Could you check a few things on this model? Use its own coordinates, in mm. A direction names the side the tool comes from. Round coordinates to 2 decimals unless told otherwise and drop trailing zeros. Loops run counter-clockwise (first coordinate to the right, second up) from the corner with the lowest first, then second, coordinate; pieces in that order, holes last. Notation, with made-up numbers: (86.25, 83.25) -> (122.25, 83.25) arc R17 ccw to (122.25, 89.25) -> close; hole circle Ø1 at (24.25, -36). An arc over 180 degrees is marked (long way). One line per item, written item: value.
from build123d import *

# Parameters (mm, degrees)
F1_DEPTH = 25.4
F2_R     = 4.7625
F3_DEPTH = 12.701
F5_DEPTH = 12.7
F6_R     = 1.5875
F7_DEPTH = 38.101
F8_R     = 5.08
F9_R     = 12.7
F10_R    = 2.032


with BuildPart() as f1:
    # F0 (on Front) → F1 (new body, symmetric)
    with BuildSketch(Plane.XZ):
        with BuildLine():
            Line((-53.975, 0), (-31.75, 0))
            ThreePointArc((-31.75, 0), (-31.0802754355, 6.4868311871), (-29.099355663, 12.7))
            Line((-29.099355663, 12.7), (-53.975, 12.7))
            Line((-53.975, 12.7), (-53.975, 0))
        make_face()
        with BuildLine():
            ThreePointArc((29.099355663, 12.7), (31.0802754355, 6.4868311871), (31.75, 0))
            Line((31.75, 0), (53.975, 0))
            Line((53.975, 0), (53.975, 38.1))
            Line((53.975, 38.1), (41.275, 38.1))
            Line((41.275, 38.1), (41.275, 12.7))
            Line((41.275, 12.7), (29.099355663, 12.7))
        make_face()
        with BuildLine():
            ThreePointArc((-14.1990316571, 12.7), (0, 19.05), (14.1990316571, 12.7))
            Line((14.1990316571, 12.7), (29.099355663, 12.7))
            ThreePointArc((29.099355663, 12.7), (0, 31.75), (-29.099355663, 12.7))
            Line((-29.099355663, 12.7), (-14.1990316571, 12.7))
        make_face()
        with BuildLine():
            ThreePointArc((14.1990316571, 12.7), (17.7959834382, 6.7974608102), (19.05, 0))
            Line((19.05, 0), (31.75, 0))
            ThreePointArc((31.75, 0), (31.0802754355, 6.4868311871), (29.099355663, 12.7))
            Line((29.099355663, 12.7), (14.1990316571, 12.7))
        make_face()
        with BuildLine():
            Line((-31.75, 0), (-19.05, 0))
            ThreePointArc((-19.05, 0), (-17.7959834382, 6.7974608102), (-14.1990316571, 12.7))
            Line((-14.1990316571, 12.7), (-29.099355663, 12.7))
            ThreePointArc((-29.099355663, 12.7), (-31.0802754355, 6.4868311871), (-31.75, 0))
        make_face()
    extrude(amount=F1_DEPTH, both=True)

    # F2 (on face) → F3 (cut, through all)
    with BuildSketch(Plane.XY.offset(12.7)):
        with Locations((-41.275, 11.3)):
            Circle(F2_R)
        with Locations((-41.275, -11.3)):
            Circle(F2_R)
    extrude(amount=-F3_DEPTH, mode=Mode.SUBTRACT)

    # F4 (on face) → F5 (cut, through all)
    with BuildSketch(Plane.YZ.offset(53.975)):
        with BuildLine():
            Line((6.5, 38.1), (-6.5, 38.1))
            Line((-6.5, 38.1), (-6.5, 25))
            ThreePointArc((-6.5, 25), (0, 31.5), (6.5, 25))
            Line((6.5, 25), (6.5, 38.1))
        make_face()
        with BuildLine():
            ThreePointArc((6.5, 25), (0, 31.5), (-6.5, 25))
            Line((-6.5, 25), (6.5, 25))
        make_face()
        with BuildLine():
            Line((6.5, 25), (-6.5, 25))
            ThreePointArc((-6.5, 25), (0, 18.5), (6.5, 25))
        make_face()
    extrude(amount=-F5_DEPTH, mode=Mode.SUBTRACT)

    # F6 (on face) → F7 (cut, through all)
    with BuildSketch(Plane(origin=(0, 0, 0), x_dir=(1, 0, 0), z_dir=(0, 0, -1))):
        Circle(F6_R)
    extrude(amount=-F7_DEPTH, mode=Mode.SUBTRACT)

    # F8
    f8_edges = [f1.edges().sort_by_distance(p)[0] for p in [
        (47.625, -25.4, 38.1),
        (47.625, 25.4, 38.1),
        (29.099356, 0, 12.7),
        (41.275, 0, 12.7),
        (-29.099356, 0, 12.7),
    ]]
    fillet(f8_edges, radius=F8_R)

    # F9
    f9_edges = [f1.edges().sort_by_distance(p)[0] for p in [
        (-53.975, 25.4, 6.35),
        (-53.975, -25.4, 6.35),
    ]]
    fillet(f9_edges, radius=F9_R)

    # F10
    f10_edges = [f1.edges().sort_by_distance(p)[0] for p in [
        (-36.7645, -25.4, 12.7),
    ]]
    fillet(f10_edges, radius=F10_R)


solid = f1.part
(1) If we section it at D-D, the plane y = 4: Please give me the cut outline in (x, z) (3 decimals).
Recorded:
outline: (-53.975, 0) -> (-19.05, 0) arc R19.05 cw to (19.05, 0) -> (53.975, 0) -> (53.975, 19.877) -> (41.275, 19.877) -> (41.275, 17.78) arc R5.08 cw to (36.195, 12.7) -> (32.254, 12.7) arc R5.08 cw to (27.805, 15.328) arc R31.75 ccw to (-27.805, 15.328) arc R5.08 cw to (-32.254, 12.7) -> (-51.943, 12.7) arc R2.032 ccw to (-53.975, 10.668) -> close
(2) If we section it at B-B, the plane z = 4: Please give me the cut outline in (x, y) (1 decimal), then the cut area to 3 significant figures.
Recorded:
outline: (-54, -12.7) arc R12.7 ccw to (-41.3, -25.4) -> (-18.6, -25.4) -> (-18.6, 25.4) -> (-41.3, 25.4) arc R12.7 ccw to (-54, 12.7) -> close; (18.6, -25.4) -> (54, -25.4) -> (54, 25.4) -> (18.6, 25.4) -> close; hole circle Ø9.5 at (-41.3, -11.3); hole circle Ø9.5 at (-41.3, 11.3)
area: 3,380 mm²
(3) If we section it at C-C, the plane x = 0: Please give me the cut outline in (y, z).
Recorded:
outline: (-25.4, 19.05) -> (-1.59, 19.05) -> (-1.59, 31.75) -> (-23.37, 31.75) arc R2.03 ccw to (-25.4, 29.72) -> close; (1.59, 19.05) -> (25.4, 19.05) -> (25.4, 29.72) arc R2.03 ccw to (23.37, 31.75) -> (1.59, 31.75) -> close
(4) Thinking about a two-plate mould opening in Y: for faces 1 (the face through (48, 6.5, 31)), 2 (the face through (48.566, -23.951, 36.572)), 3 (the face through (41.275, -6, 21)), 4 (the face through (48.566, 23.951, 36.572)), which applies, released by +Y, released by -Y, zero draft, split by the parting line, or undercut?
Recorded:
face 1: undercut
face 2: released by -Y
face 3: zero draft
face 4: released by +Y
(5) I'm going to push flat-ended pins straight in: pin 1 Ø21.5 at (x, y) = (-40, 4.5) entering from +Z; pin 2 Ø10 at (y, z) = (-19, 19) entering from -X; pin 3 Ø1.5 at (x, z) = (40.5, 15.5) entering from +Y. Where does each tip first touch, or does it pass through?
Recorded:
pin 1: z = 13.68
pin 2: x = -28.86
pin 3: y = 24.75
(6) If I drill on L1, parallel to Y at x = -40, z = 2; L2, parallel to X at y = -8, z = 8.5 (3 decimals); L3, parallel to X at y = 12, z = 8.5 (3 decimals), over which ranges is the centre line in solid material (lowest first)?
Recorded:
L1: -25.4 to -15.89, -6.71 to 6.71, 15.89 to 25.4
L2: -53.975 to -44.709, -37.841 to -17.049, 17.049 to 53.975
L3: -53.975 to -45.986, -36.564 to -17.049, 17.049 to 53.975
(7) For faces 5 (the face through (-36.7, 24.79, 12.12)), 6 (the face through (-36.83, -24.79, 12.12)), 7 (the face through (34.25, 24.79, 12.12)), 8 (the face through (39.8, -0.3, 14.2)), which set-ups out of +Z, -Z, +X, -X, +Y, -Y let a thin tool reach every point of the face, with its end or its side?
Recorded:
face 5: +Z, -X, +Y
face 6: +Z, -X, -Y
face 7: +Z, +Y
face 8: +Z, +Y, -Y
